Drawing for the job (mm, zero at the part's lowest x, y, z). A direction names the side the tool comes from. Round coordinates to 2 decimals unless told otherwise and drop trailing zeros. Loops run counter-clockwise (first coordinate to the right, second up) from the corner with the lowest first, then second, coordinate; pieces in that order, holes last. Notation, with made-up numbers: M 83.5,65 L 142.5,65 A34 ccw 142.5,96 Z; hole C -36.75,46.5 d1. An arc over 180 degrees is marked long. Answer in a Markdown table with one row per item.
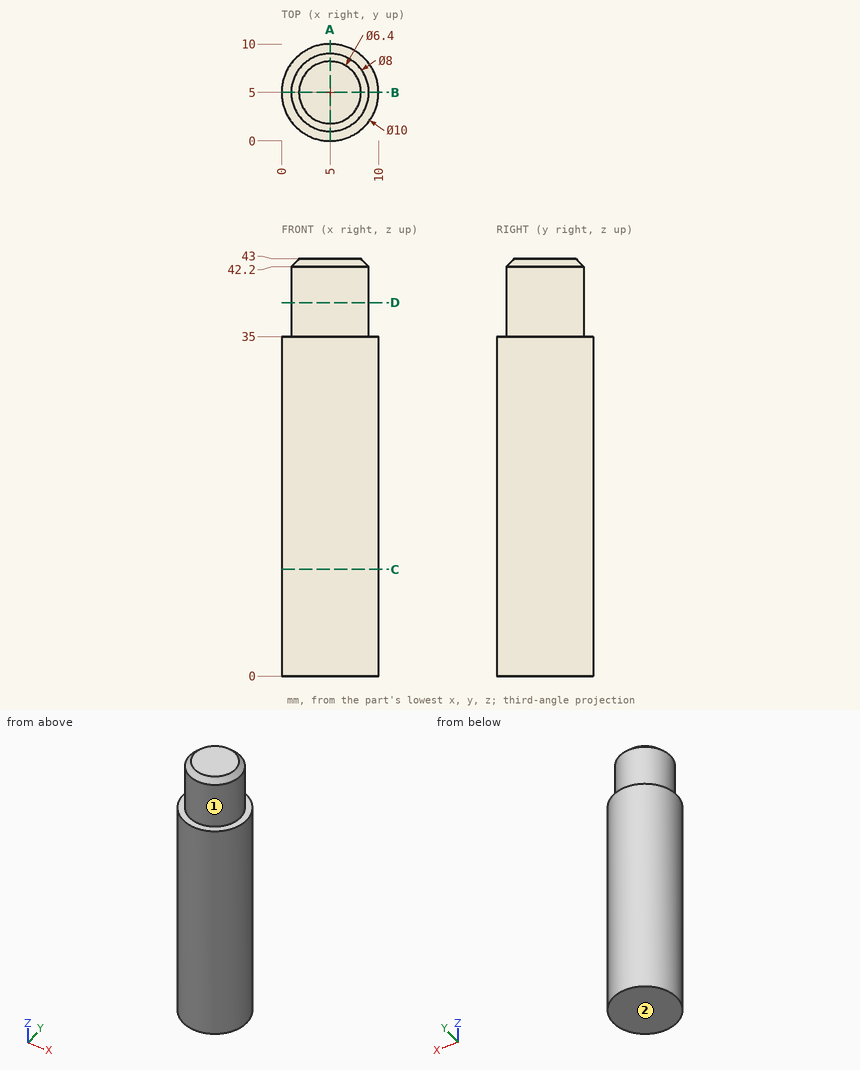
1. Saw through at C-C (z = 11). Write the cut outline in (x, y).
Verdict:
| item | result |
|---|---|
| outline | C 5,5 d10 |
2. Saw through at D-D (z = 38.5). Write the cut outline in (x, y), and give its area (3 significant figures).
Verdict:
| item | result |
|---|---|
| outline | C 5,5 d8 |
| area | 50.3 mm² |
3. Wall check: probe 1 along Y at (x, z) = (8, 20); probe 2 along Z at (x, y) = (7.25, 9). Give the ranges that are in metal, low to high.
Verdict:
| item | result |
|---|---|
| probe 1 | y = 1 to 9 |
| probe 2 | z = 0 to 35 |
4. Pin check, flat tips, straight feed: pin 1 (5 mm diameter, centred on x = 8.5, z = 35.5, fed in from +Y); pin 2 (1 mm diameter, centred on y = 8, z = 8.5, fed in from +X); pin 3 (1 mm diameter, centred on y = 3, z = 31.5, fed in from -X). Stop position of each tip, or through.
Verdict:
| item | result |
|---|---|
| pin 1 | stops at y = 9.89 |
| pin 2 | stops at x = 9.33 |
| pin 3 | stops at x = 0.23 |
5. Saw through at A-A (x = 5). Write the cut outline in (y, z).
Verdict:
| item | result |
|---|---|
| outline | M 0,0 L 10,0 L 10,35 L 9,35 L 9,42.2 L 8.2,43 L 1.8,43 L 1,42.2 L 1,35 L 0,35 Z |
6. Tool access for the marked faces 1 and 2: list every direction of +Z, -Z, +X, -X, +Y, -Y with a clear straight run to the whole face (end or side of a thin tool).
Verdict:
| item | result |
|---|---|
| face 1 | +Z |
| face 2 | -Z, +X, -X, +Y, -Y |
